Design review of the part built by this model. Coordinates are the model's own, in mm. A direction names the side the tool comes from. Coordinates: 2 decimals unless noted, no trailing zeros. Loops run counter-clockwise (first coordinate to the right, second up) from the corner with the lowest first, then second, coordinate; pieces in that order, holes last. Notation, with made-up numbers: M 10.5,-38.5 L 19.5,-38.5 A14 ccw 19.5,-33.5 Z; hole C 34,-13.75 d9. An arc over 180 degrees is marked long. One line per item, written item: value.
```python
from build123d import *

# Parameters (mm, degrees)
BOSS_EXTRUDE1_DEPTH = 2
FILLET2_R           = 5
FILLET1_R           = 0.5
SKETCH2_W           = 3
SKETCH2_H           = 7
CUT_EXTRUDE1_DEPTH  = 10
CHAMFER1_SIZE       = 0.5


with BuildPart() as part:
    # Sketch1 → Boss-Extrude1 (new body)
    with BuildSketch(Plane(origin=(0, 0, 0), x_dir=(1, 0, 0), z_dir=(0, 1, 0))):
        with BuildLine():
            Line((0, 5.1), (3, 5.1))
            Line((3, 5.1), (3, 11.9))
            Line((3, 11.9), (-17, 11.9))
            ThreePointArc((-17, 11.9), (-21.929141392, 0), (-17, -11.9))
            Line((-17, -11.9), (3, -11.9))
            Line((3, -11.9), (3, -5.1))
            Line((3, -5.1), (0, -5.1))
            ThreePointArc((0, -5.1), (-5.1, 0), (0, 5.1))
        make_face()
    extrude(amount=BOSS_EXTRUDE1_DEPTH)

    # Fillet2
    fillet2_edges = [part.edges().sort_by_distance(p)[0] for p in [
        (-17, 1, 11.9),
        (-17, 1, -11.9),
    ]]
    fillet(fillet2_edges, radius=FILLET2_R)

    # Fillet1
    fillet1_edges = [part.edges().sort_by_distance(p)[0] for p in [
        (-5.854128071, 2, -11.9),
        (-5.854128071, 0, 11.9),
        (-5.854128071, 2, 11.9),
        (-21.929141392, 0, 0),
        (-16.990510437, 0, -11.348743118),
        (-16.990510437, 0, 11.348743118),
        (-21.929141392, 2, 0),
        (-16.990510437, 2, -11.348743118),
        (-16.990510437, 2, 11.348743118),
        (-5.854128071, 0, -11.9),
    ]]
    fillet(fillet1_edges, radius=FILLET1_R)

    # Sketch2 → Cut-Extrude1 (cut)
    with BuildSketch(Plane(origin=(0, 2, 0), x_dir=(1, 0, 0), z_dir=(0, 1, 0))):
        with Locations((-3.5, 11.4)):
            Rectangle(SKETCH2_W, SKETCH2_H)
        with Locations((-3.5, -11.4)):
            Rectangle(SKETCH2_W, SKETCH2_H)
    extrude(amount=-CUT_EXTRUDE1_DEPTH, mode=Mode.SUBTRACT)

    # Chamfer1
    chamfer1_edges = [part.edges().sort_by_distance(p)[0] for p in [
        (-2, 1, -7.9),
        (-5, 1, -7.9),
        (-5, 1, 7.9),
        (-2, 1, 7.9),
    ]]
    chamfer(chamfer1_edges, length=CHAMFER1_SIZE)


solid = part.part
```
(1) We need section B-B on x = -4. State the section outline as (y, z) points.
Reply:
outline: M 0,-7.9 L 2,-7.9 L 2,-3.16 L 0,-3.16 Z; M 0,3.16 L 2,3.16 L 2,7.9 L 0,7.9 Z
(2) We need section A-A on y = 1. State the section outline as (x, z) points, then the cut area to 3 significant figures.
Reply:
outline: M -18.77,-9.82 A5 ccw -14.71,-11.9 L -5,-11.9 L -5,-8.4 L -4.5,-7.9 L -2.5,-7.9 L -2,-8.4 L -2,-11.9 L 3,-11.9 L 3,-5.1 L 0,-5.1 A5.1 cw 0,5.1 L 3,5.1 L 3,11.9 L -2,11.9 L -2,8.4 L -2.5,7.9 L -4.5,7.9 L -5,8.4 L -5,11.9 L -14.71,11.9 A5 ccw -18.77,9.82 A16.83 ccw Z
area: 460 mm2
(3) We need section C-C on z = 0. State the section outline as (x, y) points.
Reply:
outline: M -21.93,0.5 A0.5 ccw -21.43,0 L -5.1,0 L -5.1,2 L -21.43,2 A0.5 ccw -21.93,1.5 Z
(4) To check wall thickness, follow line 1 along Z through (x, y) = (0, 1.2); line 2 along X through (y, z) = (0.55, 9.75); line 3 along X through (y, z) = (0.95, 10). State the ranges of each line that lie inside material, in increasing order. Write a range as [from, to].
Reply:
line 1: z = [-11.9, -5.1], [5.1, 11.9]
line 2: x = [-18.82, -5], [-2, 3]
line 3: x = [-18.63, -5], [-2, 3]
(5) Insertion check: pin 1 (0.6 mm diameter, centred on y = 1.5, z = -10.5, fed in from -X). The pin has a flat end and moves straight along its axis. Give the tip position at first contact, or say it passes through.
Reply:
pin 1: stops at x = -18.46
(6) Tool access review of faces 5 (the flat face through (-4, 1, 7.9)), 6 (the cylindrical face through (-17.02, 1.007, 11.334)), 7 (the flat face through (2, 1, 5.1)), 8 (the flat face through (-4, 1, -7.9)): name each direction out of +Z, -Z, +X, -X, +Y, -Y from which nothing blocks a thin tool from reaching the whole face with its end or side.
Reply:
face 5: +Z, +Y, -Y
face 6: +Z, -X, +Y, -Y
face 7: +X, +Y, -Y
face 8: -Z, +Y, -Y
(7) Mouldability with a two-part tool opening along Z and no side actions: class faces 1 (the flat face through (-2, 1, -10)), 2 (the flat face through (-10, 1, 11.9)), 3 (the flat face through (-10, 1, -11.9)), 4 (the cylindrical face through (-5.1, 1, 0.1)) as released by +Z, released by -Z, zero draft, split by the parting line, or undercut.
Reply:
face 1: zero draft
face 2: released by +Z
face 3: released by -Z
face 4: undercut
